Can you work these out from the model? Positions are in its coordinate system, mm. Face numbers are marked on the shaded views. A direction names the side the tool comes from. Give positions to 0.01 mm unless a question says otherwise; leave off trailing zeros. Loops run counter-clockwise (first coordinate to the right, second up) from the corner with the lowest first, then second, coordinate; pieces in that order, holes last. Notation, with made-up numbers: M -6.5,21 L 51.5,21 A14 cw 51.5,26 Z; hole C 44.25,53 d4. An arc over 180 degrees is marked long. Use CSV: the item, a comma, the result in double quotes.
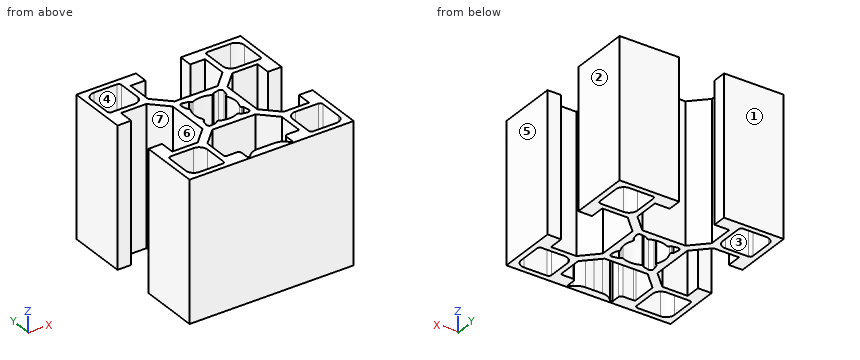
from build123d import *

# Parameters (mm, degrees)
EXTRUSION3_DEPTH = 25.4


with BuildPart() as part:
    # Sketch1 → Extrusion3 (new body)
    with BuildSketch(Plane.XY):
        Polygon((-15.000000011, 14.999999975), (-14.999999998, 4.099998455), (-12.499999998, 4.099998455), (-12.499999998, 6.799995405), (-7.860655598, 6.799995405), (-5.002158168, 3.941497975), (-5.002158168, -3.941498015), (-7.860655598, -6.799995445), (-12.499999998, -6.799995445), (-12.499999998, -4.099998495), (-14.999999998, -4.099998495), (-14.999999998, -15.000000015), (14.999999982, -15.000000015), (14.999999982, -4.099998495), (12.499999982, -4.099998495), (12.499999982, -6.799995445), (7.860655582, -6.799995445), (5.002158152, -3.941498015), (5.002158152, 3.941497975), (7.860655582, 6.799995405), (12.499999982, 6.799995405), (12.499999982, 4.099998455), (14.999999982, 4.099998455), (14.999999982, 14.999999975), (4.099998462, 14.999999975), (4.099998462, 12.499999975), (6.799995412, 12.499999975), (6.799995412, 7.860655575), (3.941497982, 5.002158145), (-3.941498008, 5.002158145), (-6.799995438, 7.860655575), (-6.799995438, 12.499999975), (-4.099998488, 12.499999975), (-4.099998488, 14.999999975), align=None)
        with BuildLine():
            Line((13.499999982, 7.799995395), (9.299995412, 7.799995395))
            ThreePointArc((9.299995412, 7.799995395), (8.239335242, 8.239335225), (7.799995412, 9.299995395))
            Line((7.799995412, 9.299995395), (7.799995412, 13.499999965))
            ThreePointArc((7.799995412, 13.499999965), (7.946442022, 13.853553355), (8.299995412, 13.999999965))
            Line((8.299995412, 13.999999965), (12.499999982, 13.999999965))
            ThreePointArc((12.499999982, 13.999999965), (13.560660152, 13.560660135), (13.999999982, 12.499999965))
            Line((13.999999982, 12.499999965), (13.999999982, 8.299995395))
            ThreePointArc((13.999999982, 8.299995395), (13.853553372, 7.946442005), (13.499999982, 7.799995395))
        make_face(mode=Mode.SUBTRACT)
        with BuildLine():
            Line((-7.799995428, 13.499999965), (-7.799995428, 9.299995395))
            ThreePointArc((-7.799995428, 9.299995395), (-8.239335258, 8.239335225), (-9.299995428, 7.799995395))
            Line((-9.299995428, 7.799995395), (-13.499999998, 7.799995395))
            ThreePointArc((-13.499999998, 7.799995395), (-13.853553388, 7.946442005), (-13.999999998, 8.299995395))
            Line((-13.999999998, 8.299995395), (-13.999999998, 12.499999965))
            ThreePointArc((-13.999999998, 12.499999965), (-13.560660168, 13.560660135), (-12.499999998, 13.999999965))
            Line((-12.499999998, 13.999999965), (-8.299995428, 13.999999965))
            ThreePointArc((-8.299995428, 13.999999965), (-7.946442038, 13.853553355), (-7.799995428, 13.499999965))
        make_face(mode=Mode.SUBTRACT)
        with BuildLine():
            Line((7.799995412, -13.500000015), (7.799995412, -9.299995445))
            ThreePointArc((7.799995412, -9.299995445), (8.239335242, -8.239335275), (9.299995412, -7.799995445))
            Line((9.299995412, -7.799995445), (13.499999982, -7.799995445))
            ThreePointArc((13.499999982, -7.799995445), (13.853553372, -7.946442055), (13.999999982, -8.299995445))
            Line((13.999999982, -8.299995445), (13.999999982, -12.500000015))
            ThreePointArc((13.999999982, -12.500000015), (13.560660152, -13.560660185), (12.499999982, -14.000000015))
            Line((12.499999982, -14.000000015), (8.299995412, -14.000000015))
            ThreePointArc((8.299995412, -14.000000015), (7.946442022, -13.853553405), (7.799995412, -13.500000015))
        make_face(mode=Mode.SUBTRACT)
        with BuildLine():
            Line((-13.499999998, -7.799995445), (-9.299995428, -7.799995445))
            ThreePointArc((-9.299995428, -7.799995445), (-8.239335258, -8.239335275), (-7.799995428, -9.299995445))
            Line((-7.799995428, -9.299995445), (-7.799995428, -13.500000015))
            ThreePointArc((-7.799995428, -13.500000015), (-7.946442038, -13.853553405), (-8.299995428, -14.000000015))
            Line((-8.299995428, -14.000000015), (-12.499999998, -14.000000015))
            ThreePointArc((-12.499999998, -14.000000015), (-13.560660168, -13.560660185), (-13.999999998, -12.500000015))
            Line((-13.999999998, -12.500000015), (-13.999999998, -8.299995445))
            ThreePointArc((-13.999999998, -8.299995445), (-13.853553388, -7.946442055), (-13.499999998, -7.799995445))
        make_face(mode=Mode.SUBTRACT)
        with BuildLine():
            Line((-3.285876608, 3.878886835), (-2.243073548, 3.657287075))
            Line((-2.243073548, 3.657287075), (-2.005134008, 3.419347535))
            ThreePointArc((-2.005134008, 3.419347535), (-1.841800007, 3.335474925), (-1.660187018, 3.362481085))
            ThreePointArc((-1.660187018, 3.362481085), (-2.3e-08, 3.749999985), (1.660186972, 3.362481085))
            ThreePointArc((1.660186972, 3.362481085), (1.841799961, 3.335474925), (2.005133962, 3.419347535))
            Line((2.005133962, 3.419347535), (2.243073502, 3.657287075))
            Line((2.243073502, 3.657287075), (3.285876562, 3.878886835))
            ThreePointArc((3.285876562, 3.878886835), (3.743361172, 3.743361195), (3.878886812, 3.285876585))
            Line((3.878886812, 3.285876585), (3.657287052, 2.243073525))
            Line((3.657287052, 2.243073525), (3.419347512, 2.005133985))
            ThreePointArc((3.419347512, 2.005133985), (3.335474902, 1.841799984), (3.362481062, 1.660186995))
            ThreePointArc((3.362481062, 1.660186995), (3.749999954, -2e-09), (3.362481062, -1.660186995))
            ThreePointArc((3.362481062, -1.660186995), (3.335474902, -1.841799984), (3.419347512, -2.005133985))
            Line((3.419347512, -2.005133985), (3.657287052, -2.243073525))
            Line((3.657287052, -2.243073525), (3.878886812, -3.285876585))
            ThreePointArc((3.878886812, -3.285876585), (3.743361172, -3.743361195), (3.285876562, -3.878886835))
            Line((3.285876562, -3.878886835), (2.243073502, -3.657287075))
            Line((2.243073502, -3.657287075), (2.005133962, -3.419347535))
            ThreePointArc((2.005133962, -3.419347535), (1.841799961, -3.335474925), (1.660186972, -3.362481085))
            ThreePointArc((1.660186972, -3.362481085), (-2.3e-08, -3.74999999), (-1.660187018, -3.362481085))
            ThreePointArc((-1.660187018, -3.362481085), (-1.841800007, -3.335474925), (-2.005134008, -3.419347535))
            Line((-2.005134008, -3.419347535), (-2.243073548, -3.657287075))
            Line((-2.243073548, -3.657287075), (-3.285876608, -3.878886835))
            ThreePointArc((-3.285876608, -3.878886835), (-3.743361218, -3.743361195), (-3.878886858, -3.285876585))
            Line((-3.878886858, -3.285876585), (-3.657287098, -2.243073525))
            Line((-3.657287098, -2.243073525), (-3.419347558, -2.005133985))
            ThreePointArc((-3.419347558, -2.005133985), (-3.335474948, -1.841799984), (-3.362481108, -1.660186995))
            ThreePointArc((-3.362481108, -1.660186995), (-3.750000021, -2e-09), (-3.362481108, 1.660186995))
            ThreePointArc((-3.362481108, 1.660186995), (-3.335474948, 1.841799984), (-3.419347558, 2.005133985))
            Line((-3.419347558, 2.005133985), (-3.657287098, 2.243073525))
            Line((-3.657287098, 2.243073525), (-3.878886858, 3.285876585))
            ThreePointArc((-3.878886858, 3.285876585), (-3.743361218, 3.743361195), (-3.285876608, 3.878886835))
        make_face(mode=Mode.SUBTRACT)
        with BuildLine():
            Line((-6.799995418, -7.860655625), (-3.941497998, -5.002158195))
            Line((-3.941497998, -5.002158195), (3.941497992, -5.002158195))
            Line((3.941497992, -5.002158195), (6.799995422, -7.860655625))
            Line((6.799995422, -7.860655625), (6.799995422, -12.199996975))
            ThreePointArc((6.799995422, -12.199996975), (6.712130925, -12.412130132), (6.500000002, -12.500000025))
            Line((6.500000002, -12.500000025), (4.599998472, -12.500000025))
            ThreePointArc((4.599998472, -12.500000025), (4.246445082, -12.646446635), (4.099998472, -13.000000025))
            Line((4.099998472, -13.000000025), (4.099998472, -14.600000025))
            Line((4.099998472, -14.600000025), (3.699990832, -14.600000025))
            Line((3.699990832, -14.600000025), (3.332307072, -14.232291555))
            ThreePointArc((3.332307072, -14.232291555), (2.521228054, -13.690316336), (1.564480612, -13.499999115))
            Line((1.564480612, -13.499999115), (-5.8e-08, -13.499999185))
            Line((-5.8e-08, -13.499999185), (-1.564449118, -13.499999135))
            ThreePointArc((-1.564449118, -13.499999135), (-2.521158976, -13.690300794), (-3.332218038, -14.232234065))
            Line((-3.332218038, -14.232234065), (-3.699983218, -14.600000025))
            Line((-3.699983218, -14.600000025), (-4.099998468, -14.600000025))
            Line((-4.099998468, -14.600000025), (-4.099998468, -13.000000025))
            ThreePointArc((-4.099998468, -13.000000025), (-4.246445078, -12.646446635), (-4.599998468, -12.500000025))
            Line((-4.599998468, -12.500000025), (-6.499999998, -12.500000025))
            ThreePointArc((-6.499999998, -12.500000025), (-6.712130926, -12.412130137), (-6.799995418, -12.199996975))
            Line((-6.799995418, -12.199996975), (-6.799995418, -7.860655625))
        make_face(mode=Mode.SUBTRACT)
    extrude(amount=EXTRUSION3_DEPTH)


solid = part.part
Q1. I want a section at D-D, the plane z = 9.25. State how many separate pieces and enclosed holes the cut face has, then the cut area to 3 significant figures.
Model answer:
separate pieces,"1"
enclosed holes,"6"
area,"250 mm2"
Q2. If we mould it in two halves opening along Y, with no side actions, what happens to the marked faces 1, 2, 3 and 4? For each: released by +Y, released by -Y, zero draft, split by the parting line, or undercut.
Model answer:
face 1,"released by +Y"
face 2,"zero draft"
face 3,"undercut"
face 4,"undercut"
Q3. I want a section at B-B, the plane x = 0.75. Please give me the cut outline in (y, z).
Model answer:
outline,"M -15,0 L -13.5,0 L -13.5,25.4 L -15,25.4 Z; M -5,0 L -3.67,0 L -3.67,25.4 L -5,25.4 Z; M 3.67,0 L 5,0 L 5,25.4 L 3.67,25.4 Z"
Q4. I'm going to push flat-ended pins straight in: P1, Ø8.5, axis at y = -0.5, z = 17.5, coming from the -X side; P2, Ø2.5, axis at y = 0.5, z = 16, coming from the +X side. Where does each tip first touch, or does it pass through?
Model answer:
P1,"x = -15"
P2,"x = 5"
Q5. I want a section at C-C, the plane x = -5.5. Please give me the cut outline in (y, z).
Model answer:
outline,"M -15,0 L -12.5,0 L -12.5,25.4 L -15,25.4 Z; M -6.56,0 L -4.44,0 L -4.44,25.4 L -6.56,25.4 Z; M 4.44,0 L 6.56,0 L 6.56,25.4 L 4.44,25.4 Z; M 12.5,0 L 15,0 L 15,25.4 L 12.5,25.4 Z"
Q6. I want a section at A-A, the plane y = -9.75. Please give me the cut outline in (x, z), then the cut area to 3 significant figures.
Model answer:
outline,"M -15,0 L -14,0 L -14,25.4 L -15,25.4 Z; M -7.8,0 L -6.8,0 L -6.8,25.4 L -7.8,25.4 Z; M 6.8,0 L 7.8,0 L 7.8,25.4 L 6.8,25.4 Z; M 14,0 L 15,0 L 15,25.4 L 14,25.4 Z"
area,"102 mm2"
Q7. For the marked faces 5, 6 and 7, which set-ups out of +Z, -Z, +X, -X, +Y, -Y let a thin tool reach every point of the face, with its end or its side?
Model answer:
face 5,"+Z, -Z, +X, +Y, -Y"
face 6,"+Z, -Z, -X"
face 7,"+Z, -Z"
Q8. Please list where these lines run through material, in increasing order: L1, parallel to X at y = -12.25, z = 16.25; L2, parallel to X at y = -12.75, z = 7. Write a range as from..to.
Model answer:
L1,"-15..-14, -7.8..-6.8, 6.8..7.8, 14..15"
L2,"-15..-13.98, -7.8..-4.17, 4.17..7.8, 13.98..15"
